```python
from build123d import *

# Parameters (mm, degrees)
SKETCH1_W           = 208
SKETCH1_H           = 46
BOSS_EXTRUDE1_DEPTH = 14
SKETCH2_R           = 6
BOSS_EXTRUDE2_DEPTH = 54
SKETCH3_W           = 28
SKETCH3_H           = 28
CUT_EXTRUDE1_DEPTH  = 12
CUT_EXTRUDE2_START  = -12
SKETCH4_R           = 6
CUT_EXTRUDE2_DEPTH  = 12
SKETCH5_W           = 195
SKETCH5_H           = 33
CUT_EXTRUDE3_DEPTH  = 2
CUT_EXTRUDE4_DEPTH  = 133.4990566
SKETCH8_R           = 4
CUT_EXTRUDE7_DEPTH  = 126.303631232
SKETCH8_2_R         = 4
BOSS_EXTRUDE3_DEPTH = 16


with BuildPart() as part:
    # Sketch1 → Boss-Extrude1 (new body)
    with BuildSketch(Plane(origin=(0, 0, 0), x_dir=(1, 0, 0), z_dir=(0, 1, 0))):
        Rectangle(SKETCH1_W, SKETCH1_H)
        with BuildLine():
            Line((-85, 6), (-77, 6))
            ThreePointArc((-77, 6), (-71, 0), (-77, -6))
            Line((-77, -6), (-85, -6))
            ThreePointArc((-85, -6), (-91, 0), (-85, 6))
        make_face(mode=Mode.SUBTRACT)
        with BuildLine():
            Line((85, -6), (77, -6))
            ThreePointArc((77, -6), (71, 0), (77, 6))
            Line((77, 6), (85, 6))
            ThreePointArc((85, 6), (91, 0), (85, -6))
        make_face(mode=Mode.SUBTRACT)
    extrude(amount=BOSS_EXTRUDE1_DEPTH)

    # Sketch2 → Boss-Extrude2 (add)
    with BuildSketch(Plane(origin=(0, 14, 0), x_dir=(1, 0, 0), z_dir=(0, 1, 0))):
        with BuildLine():
            Line((-48.856934001, 23), (48.856934001, 23))
            ThreePointArc((48.856934001, 23), (54, 0), (48.856934001, -23))
            Line((48.856934001, -23), (-48.856934001, -23))
            ThreePointArc((-48.856934001, -23), (-54, 0), (-48.856934001, 23))
        make_face()
        with Locations(Location((-39, 0, 0), (0, 0, 270))):
            Circle(SKETCH2_R, mode=Mode.SUBTRACT)
        with Locations(Location((39, 0, 0), (0, 0, 90))):
            Circle(SKETCH2_R, mode=Mode.SUBTRACT)
    extrude(amount=BOSS_EXTRUDE2_DEPTH)

    # Sketch3 → Cut-Extrude1 (cut)
    with BuildSketch(Plane.XZ):
        with Locations((-39, 0)):
            Rectangle(SKETCH3_W, SKETCH3_H)
        with Locations((39, 0)):
            Rectangle(SKETCH3_W, SKETCH3_H)
    extrude(amount=-CUT_EXTRUDE1_DEPTH, mode=Mode.SUBTRACT)

    # Sketch4 → Cut-Extrude2 (cut)
    with BuildSketch(Plane(origin=(0, 14, 0), x_dir=(1, 0, 0), z_dir=(0, 1, 0)).offset(CUT_EXTRUDE2_START)):
        with Locations(Location((39, 0, 0), (0, 0, 90))):
            Circle(SKETCH4_R)
        with Locations(Location((-39, 0, 0), (0, 0, 90))):
            Circle(SKETCH4_R)
    extrude(amount=CUT_EXTRUDE2_DEPTH, mode=Mode.SUBTRACT)

    # Sketch5 → Cut-Extrude3 (cut)
    with BuildSketch(Plane.XZ):
        Rectangle(SKETCH5_W, SKETCH5_H)
    extrude(amount=-CUT_EXTRUDE3_DEPTH, mode=Mode.SUBTRACT)

    # Sketch6 → Cut-Extrude4 (cut, through all)
    with BuildSketch(Plane.XY.offset(23)):
        with BuildLine():
            Line((-28, 68), (-28, 48))
            Line((-28, 48), (-24, 48))
            ThreePointArc((-24, 48), (-16.970562748, 31.029437252), (0, 24))
            Line((0, 24), (0, 68))
            Line((0, 68), (-28, 68))
        make_face()
        with BuildLine():
            Line((0, 68), (0, 24))
            ThreePointArc((0, 24), (16.970562748, 31.029437252), (24, 48))
            Line((24, 48), (28, 48))
            Line((28, 48), (28, 68))
            Line((28, 68), (0, 68))
        make_face()
    extrude(amount=-CUT_EXTRUDE4_DEPTH, mode=Mode.SUBTRACT)

    # Sketch8 → Cut-Extrude7 (cut, through all)
    with BuildSketch(Plane.XZ.offset(-2)):
        with Locations(Location((0, 0, 0), (0, 0, 270))):
            Circle(SKETCH8_R)
    extrude(amount=-CUT_EXTRUDE7_DEPTH, mode=Mode.SUBTRACT)

    # Sketch8_2 → Boss-Extrude3 (add)
    with BuildSketch(Plane.XZ.offset(-2)):
        with Locations(Location((0, 0, 0), (0, 0, 270))):
            Circle(SKETCH8_2_R)
    extrude(amount=-BOSS_EXTRUDE3_DEPTH)


solid = part.part
```
For this review, take the finished solid that the model builds, in its own axes (mm). A direction names the side the tool comes from. Coordinates: 2 decimals unless noted, no trailing zeros. Write each loop counter-clockwise with the first axis right and the second up, starting at its lowest first coordinate (ties: lowest second). Pieces come first, ordered by that corner, then holes. Notation, with made-up numbers: (48, 10.25) - (52, 10.25) arc R13 ccw to (52, 17.25) - close; hole circle Ø9 at (-24.75, 24.5). An arc over 180 degrees is marked (long way). Put each result on its own line as item: value.
1. For pin 1 (23 mm diameter, centred on x = 66.5, z = 9.5, fed in from +Y); pin 2 (9 mm diameter, centred on x = -1, z = -2, fed in from +Y); pin 3 (5 mm diameter, centred on y = 53, z = -12.5, fed in from -X), all flat-tipped, find the tip position at first contact; note any pin that passes through.
Values found:
pin 1: y = 14
pin 2: y = 24.64
pin 3: x = -53.07
2. Add section B-B, the plane y = 45. Give the boundary of the cut face in (x, z), then the cut area to 3 significant figures.
Values found:
outline: (-48.86, -23) - (-23.81, -23) - (-23.81, 23) - (-48.86, 23) arc R54 ccw to start; (23.81, -23) - (48.86, -23) arc R54 ccw to (48.86, 23) - (23.81, 23) - close; hole circle Ø12 at (-39, 0); hole circle Ø12 at (39, 0)
area: 2,400 mm²
3. Wall thickness on probe 1 along X at (y, z) = (22, 0); probe 2 along Z at (x, y) = (34.5, 6); probe 3 along Z at (x, y) = (-39, 53): over which ranges is each line inside the solid? List them lowest first.
Values found:
probe 1: -54 to -45, -33 to -4, 4 to 33, 45 to 54
probe 2: -23 to -14, 14 to 23
probe 3: -23 to -6, 6 to 23
4. Mouldability with a two-part tool opening along Z and no side actions: class faces 4 (the cylindrical face through (54, 41, 0)), 5 (the flat face through (-28, 58, 0)), 6 (the cylindrical face through (44.857, 39.608, 1.301)) as released by +Z, released by -Z, zero draft, split by the parting line, or undercut.
Values found:
face 4: split by the parting line
face 5: zero draft
face 6: undercut
5. Add section C-C, the plane x = 39. Give the boundary of the cut face in (y, z), then the cut area to 3 significant figures.
Values found:
outline: (0, -23) - (68, -23) - (68, -6) - (12, -6) - (12, -14) - (2, -14) - (2, -16.5) - (0, -16.5) - close; (0, 16.5) - (2, 16.5) - (2, 14) - (12, 14) - (12, 6) - (68, 6) - (68, 23) - (0, 23) - close
area: 2,110 mm²
6. Add section A-A, the plane x = -81. Give the boundary of the cut face in (y, z), then the cut area to 3 significant figures.
Values found:
outline: (0, -23) - (14, -23) - (14, -6) - (2, -6) - (2, -16.5) - (0, -16.5) - close; (0, 16.5) - (2, 16.5) - (2, 6) - (14, 6) - (14, 23) - (0, 23) - close
area: 434 mm²
7. Machinability: for faces 1 (the flat face through (39, 7, -14)), 2 (the flat face through (28, 58, 0)), 3 (the cylindrical face through (71, 8, 0)), which of the approach directions +Z, -Z, +X, -X, +Y, -Y give a long, thin tool a straight path to every point of the face, cutting with its end or side? Answer none if there is none.
Values found:
face 1: -Y
face 2: +Z, -Z, +Y
face 3: +Y, -Y
